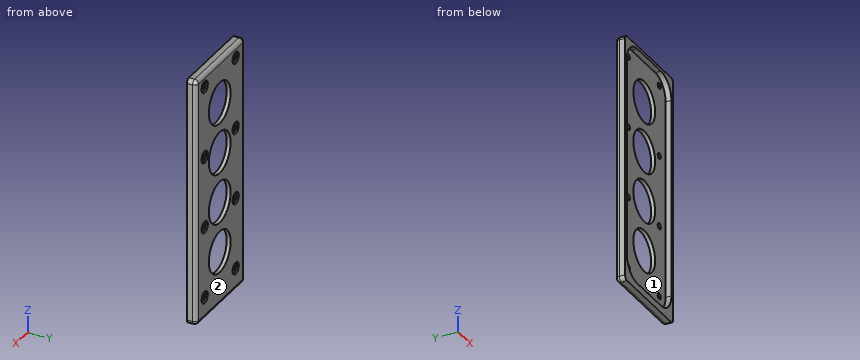
Autodesk Inventor part; units mm, degrees
ref_plane "Work Plane2 - PCB Vertical" through (0, 0, -62.5) normal (0, 0, 1) x (1, 0, 0)
ref_plane "Work Plane6 - Fond creusé" through (0, 17, 0) normal (0, 1, 0) x (-1, 0, 0)
ref_plane "Work Plane11 - Haut capteurs shields" through (0, 23.1, 0) normal (0, 1, 0) x (-1, 0, 0)
sketch "Sketch1" plane through (0, 0, 0) normal (0, 1, 0) x (-1, 0, 0)
  line L0 (2, 0) -> (102, 0)
  line L1 (104, -2) -> (104, -123)
  line L2 (102, -125) -> (2, -125)
  line L3 (0, -123) -> (0, -2)
  arc A0 (104, -2) -> (102, 0) centre (102, -2) ccw
  arc A1 (102, -125) -> (104, -123) centre (102, -123) ccw
  arc A2 (0, -123) -> (2, -125) centre (2, -123) ccw
  arc A3 (2, 0) -> (0, -2) centre (2, -2) ccw
  point P0 (0, 0)
  point P1 (104, -125)
  point P2 (0, -125)
  dimension "d0" = 104
  dimension "d1" = 125
  dimension "d2" = 2
  dimension "d3" = 2
extrude "Boîte extérieure" [suppressed]
fillet "Fillet1-Boîte extérieure" [suppressed]
ref_plane "Work Plane2 - PCB Vertical" through (0, 0, -62.5) normal (0, 0, 1) x (1, 0, 0)
ref_plane "Work Plane4 - Surface extérieure capteurs" through (0, 20.1, 0) normal (0, 1, 0) x (-1, 0, 0)
ref_plane "Work Plane6 - Fond creusé" through (0, 17, 0) normal (0, 1, 0) x (-1, 0, 0)
sketch "Sketch26" plane through (0, 20.1, 0) normal (0, 1, 0) x (-1, 0, 0)
  line L0 (16, -121) -> (36, -121)
  line L1 (47, -110) -> (47, -13)
  line L2 (36, -2) -> (16, -2)
  line L3 (5, -13) -> (5, -110)
  arc A0 (5, -110) -> (16, -121) centre (16, -110) ccw
  arc A1 (36, -121) -> (47, -110) centre (36, -110) ccw
  arc A2 (47, -13) -> (36, -2) centre (36, -13) ccw
  arc A3 (16, -2) -> (5, -13) centre (16, -13) ccw
  line L4 (0, -2) -> (0, -123)
  line L5 (0, -2) -> (0, -123)
  line L6 (104, -123) -> (104, -2)
  line L7 (2, -125) -> (102, -125)
  point P0 (0, 0)
  point P1 (47, -2)
  point P2 (47, -121)
  point P3 (5, -2)
  dimension "d158" = 42
  dimension "d159" = 119
  dimension "d160" = 11
  dimension "d161" = 5
  dimension "d186" = 4
extrude "Centreur Echantillonnage actif" [suppressed]
sketch "Sketch 22" plane through (0, 17, 0) normal (0, 1, 0) x (-1, 0, 0)
  circle A0 centre (25.1, -19.83) radius 16.5
  line L0 (99, -5) -> (99, -120)
  line L1 (9, -5) -> (99, -5)
  circle A1 centre (25.1, -47.135) radius 10.5
  circle A2 centre (25.1, -72.535) radius 10.5
  circle A3 centre (25.1, -99.84) radius 16.5
  line L2 (102, 0) -> (2, 0)
  line L3 (0, -2) -> (0, -123)
  line L4 (2, -125) -> (102, -125)
  point P0 (0, 0)
  point P1 (99, -12.0721)
  point P2 (99, -58.79)
  point P3 (16.07, -5)
  point P4 (91.93, -5)
  dimension "d124" = 33
  dimension "d126" = 14.83
  dimension "d140" = 21
  dimension "d141" = 27.305
  dimension "d142" = 21
  dimension "d143" = 25.4
  dimension "d144" = 33
  dimension "d145" = 27.305
  dimension "d196" = 73.9
  dimension "d258" = 19.83
  dimension "d259" = 25.1
  dimension "d260" = 25.16
extrude "Sensor A/Miniature or Sensoric" [suppressed]
sketch "Sketch35" plane through (0, 20.1, 0) normal (0, 1, 0) x (-1, 0, 0)
  circle A0 centre (40.5, -114) radius 1
  line L0 (47, -110) -> (47, -13)
  line L1 (16, -121) -> (36, -121)
  point P0 (0, 0)
  dimension "d235" = 2
  dimension "d244" = 6.5
  dimension "d245" = 7
extrude "Vis Centreur Chapeau" [suppressed]
pattern_linear "Rectangular Pattern3" [suppressed]
ref_plane "Work Plane10 - Chapeau ext." through (0, 25.1, 0) normal (0, 1, 0) x (-1, 0, 0)
sketch "Sketch36" plane through (0, 25.1, 0) normal (0, 1, 0) x (-1, 0, 0)
  line L0 (102, -125) -> (2, -125)
  line L1 (102, 0) -> (2, 0)
  line L2 (2.8, -125) -> (49.2, -125)
  line L3 (49.2, -125) -> (49.2, 0)
  line L4 (49.2, 0) -> (2.8, 0)
  line L5 (2.8, 0) -> (2.8, -125)
  line L6 (47, -110) -> (47, -13)
  point P0 (0, 0)
  dimension "d247" = 46.4
  dimension "d252" = 125
extrude "Chapeau" add sketch "Sketch36" against normal blind 4.9
fillet "Fillet10" radius 2 8 edges at (-49.2, 25.1, -62.5) (-26, 25.1, -125) (-49.2, 22.65, -125) (-2.8, 22.65, -125) (-2.8, 25.1, -62.5) (-2.8, 22.65, 0) (-26, 25.1, 0) (-49.2, 22.65, 0)
ref_plane "Work Plane11 - Haut capteurs shields" through (0, 23.1, 0) normal (0, 1, 0) x (-1, 0, 0)
sketch "Sketch37" plane through (0, 23.1, 0) normal (0, 1, 0) x (-1, 0, 0)
  line L0 (14.5, -1.5) -> (37.5, -1.5)
  line L1 (47.5, -11.5) -> (47.5, -111.5)
  line L2 (37.5, -121.5) -> (14.5, -121.5)
  line L3 (4.5, -111.5) -> (4.5, -11.5)
  line L4 (4.8, 0) -> (47.2, 0)
  line L5 (2.8, -123) -> (2.8, -2)
  line L6 (47.2, -125) -> (4.8, -125)
  arc A0 (4.5, -111.5) -> (14.5, -121.5) centre (14.5, -111.5) ccw
  arc A1 (37.5, -121.5) -> (47.5, -111.5) centre (37.5, -111.5) ccw
  arc A2 (47.5, -11.5) -> (37.5, -1.5) centre (37.5, -11.5) ccw
  arc A3 (14.5, -1.5) -> (4.5, -11.5) centre (14.5, -11.5) ccw
  point P0 (0, 0)
  point P1 (4.5, -1.5)
  point P2 (47.5, -121.5)
  point P3 (47.5, -1.5)
  point P4 (4.5, -121.5)
  dimension "d254" = 43
  dimension "d255" = 120
  dimension "d257" = 1.7
  dimension "d263" = 3.5
  dimension "d264" = 10
extrude "Creusement interne pour passage Centreur" cut sketch "Sketch37" against normal blind 2.9
sketch "Sketch41" plane through (0, 25.1, 0) normal (0, 1, 0) x (-1, 0, 0)
  circle A0 centre (40.5, -114) radius 1.5
  point P0 (0, 0)
  dimension "d276" = 3
extrude "Alesage de vissage chapeau" cut sketch "Sketch41" against normal blind 2
sketch "Sketch38" plane through (0, 23.1, 0) normal (0, 1, 0) x (-1, 0, 0)
  line L0 (47.2, -125) -> (4.8, -125)
  line L1 (4.8, 0) -> (47.2, 0)
  circle A0 centre (25.1, -97.935) radius 8.25
  circle A1 centre (25.1, -72.535) radius 8.25
  circle A2 centre (25.1, -47.135) radius 8.25
  point P0 (0, 0)
  point P1 (25.1, -99.84)
  point P2 (25.1, -19.83)
  point P3 (25.1, -21.735)
  dimension "d265" = 25.16
  dimension "d266" = 27.305
  dimension "d267" = 25.4
  dimension "d268" = 27.305
  dimension "d269" = 19.83
  dimension "d270" = 27.065
  dimension "d271" = 25.4
  dimension "d272" = 25.4
  dimension "d273" = 21.735
  dimension "d300" = 16.5
  dimension "d301" = 16.5
  dimension "d302" = 16.5
pattern_linear "Alesages de vissages chapeau" count 2 spacing 29.9 along (1, 0, 0) count 4 spacing 35.9 along (0, 0, 1) of "Alesage de vissage chapeau"
sketch "Sketch44" plane through (0, 25.1, 0) normal (0, 1, 0) x (-1, 0, 0)
  circle A0 centre (40.5, -114) radius 3
  point P0 (0, 0)
  dimension "d291" = 6
extrude "Epaulement tête de vis" cut sketch "Sketch44" against normal blind 1
pattern_linear "Epaulements tête de vis" count 2 spacing 29.9 along (1, 0, 0) count 4 spacing -35.9 along (0, 0, -1) of "Epaulement tête de vis"
sketch "Sketch45" plane through (0, 23.1, 0) normal (0, 1, 0) x (-1, 0, 0)
  circle A0 centre (25.1, -97.935) radius 10.5
  circle A1 centre (25.1, -72.535) radius 10.5
  circle A2 centre (25.1, -47.135) radius 10.5
  circle A3 centre (25.1, -21.735) radius 10.5
  point P0 (0, 0)
  dimension "d303" = 21
  dimension "d304" = 21
  dimension "d305" = 21
  dimension "d308" = 21
extrude "ALesages capteurs" cut sketch "Sketch45" along normal blind 2
properties part number "160409 Sensor cover A_Miniature - A_Miniature - A_Miniature - A_Miniature - R23"
Can you work these out from the model? Positions are in its coordinate system, mm. Face numbers are marked on the shaded views. Round coordinates to 2 decimals unless told otherwise and drop trailing zeros. Loops run counter-clockwise (first coordinate to the right, second up) from the corner with the lowest first, then second, coordinate; pieces in that order, holes last. Notation, with made-up numbers: M 21,58 L 37,58 A10 ccw 37,72 Z; hole C 20,18.25 d11. An arc over 180 degrees is marked long. Answer as a JSON object with one key per item and string values. Group by question number.
Q1. Imagine slicing it at C-C, the plane z = -42.2. Count the separate pieces of the cut face and the enclosed holes in it, then the cut area to 3 significant figures.
Q2. Will these pins go through, and if not, where does the flat tip stop? pin 1 (3 mm diameter, centred on x = -9.5, z = -114, fed in from +Y); pin 2 (2.5 mm diameter, centred on x = -40.5, z = -114, fed in from -Y); pin 3 (1.5 mm diameter, centred on y = 24.5, z = -31.5, fed in from +X); pin 4 (8 mm diameter, centred on x = -40.5, z = -42.2, fed in from -Y).
Q3. Imagine slicing it at B-B, the plane x = -25.1. Please give me the cut outline in (y, z) (3 decimals), then the cut area to 3 significant figures.
Q4. We'd pull the mould along X, two halves only. Please class the marked faces 1 and 2: +X half, -X half, draft (parallel to the pull), parting line (faces both ways), or undercut.
Q5. Imagine slicing it at A-A, the plane y = 22.3. Please give me the cut outline in (x, z).
Q6. Please list where these lines run through material, in increasing order: L1, parallel to Z at x = -23, y = 22.5; L2, parallel to X at y = 23.7, z = -78.1; L3, parallel to X at y = 21.6, z = -42.
Q7. Imagine slicing it at D-D, the plane z = -6.3. Please give me the cut outline in (x, y), then the cut area to 3 significant figures.
Findings:
{
 "1": {"separate pieces": "4", "enclosed holes": "0", "area": "45.9 mm2"},
 "2": {"pin 1": "stops at y = 24.1", "pin 2": "passes through", "pin 3": "stops at x = -2.91", "pin 4": "stops at y = 23.1"},
 "3": {"outline": "M 20.2,-125 L 23.1,-125 A2 ccw 25.1,-123 L 25.1,-108.435 L 23.1,-108.435 L 23.1,-121.5 L 20.2,-121.5 Z; M 20.2,-1.5 L 23.1,-1.5 L 23.1,-11.235 L 25.1,-11.235 L 25.1,-2 A2 ccw 23.1,0 L 20.2,0 Z; M 23.1,-87.435 L 25.1,-87.435 L 25.1,-83.035 L 23.1,-83.035 Z; M 23.1,-62.035 L 25.1,-62.035 L 25.1,-57.635 L 23.1,-57.635 Z; M 23.1,-36.635 L 25.1,-36.635 L 25.1,-32.235 L 23.1,-32.235 Z", "area": "94.8 mm2"},
 "4": {"face 1": "undercut", "face 2": "draft"},
 "5": {"outline": "M -49.2,-123 A2 ccw -47.2,-125 L -4.8,-125 A2 ccw -2.8,-123 L -2.8,-2 A2 ccw -4.8,0 L -47.2,0 A2 ccw -49.2,-2 Z; hole M -47.5,-111.5 A10 ccw -37.5,-121.5 L -14.5,-121.5 A10 ccw -4.5,-111.5 L -4.5,-11.5 A10 ccw -14.5,-1.5 L -37.5,-1.5 A10 ccw -47.5,-11.5 Z"},
 "6": {"L1": "z = -125 to -121.5, -1.5 to 0", "L2": "x = -49.11 to -42, -39 to -34, -16.2 to -12.1, -9.1 to -2.89", "L3": "x = -49.2 to -47.5, -4.5 to -2.8"},
 "7": {"outline": "M -49.2,20.2 L -46.04,20.2 L -46.04,23.1 L -42,23.1 L -42,24.1 L -43.5,24.1 L -43.5,25.1 L -47.2,25.1 A2 ccw -49.2,23.1 Z; M -39,23.1 L -12.1,23.1 L -12.1,24.1 L -13.6,24.1 L -13.6,25.1 L -37.5,25.1 L -37.5,24.1 L -39,24.1 Z; M -9.1,23.1 L -5.96,23.1 L -5.96,20.2 L -2.8,20.2 L -2.8,23.1 A2 ccw -4.8,25.1 L -7.6,25.1 L -7.6,24.1 L -9.1,24.1 Z", "area": "91.4 mm2"}
}
